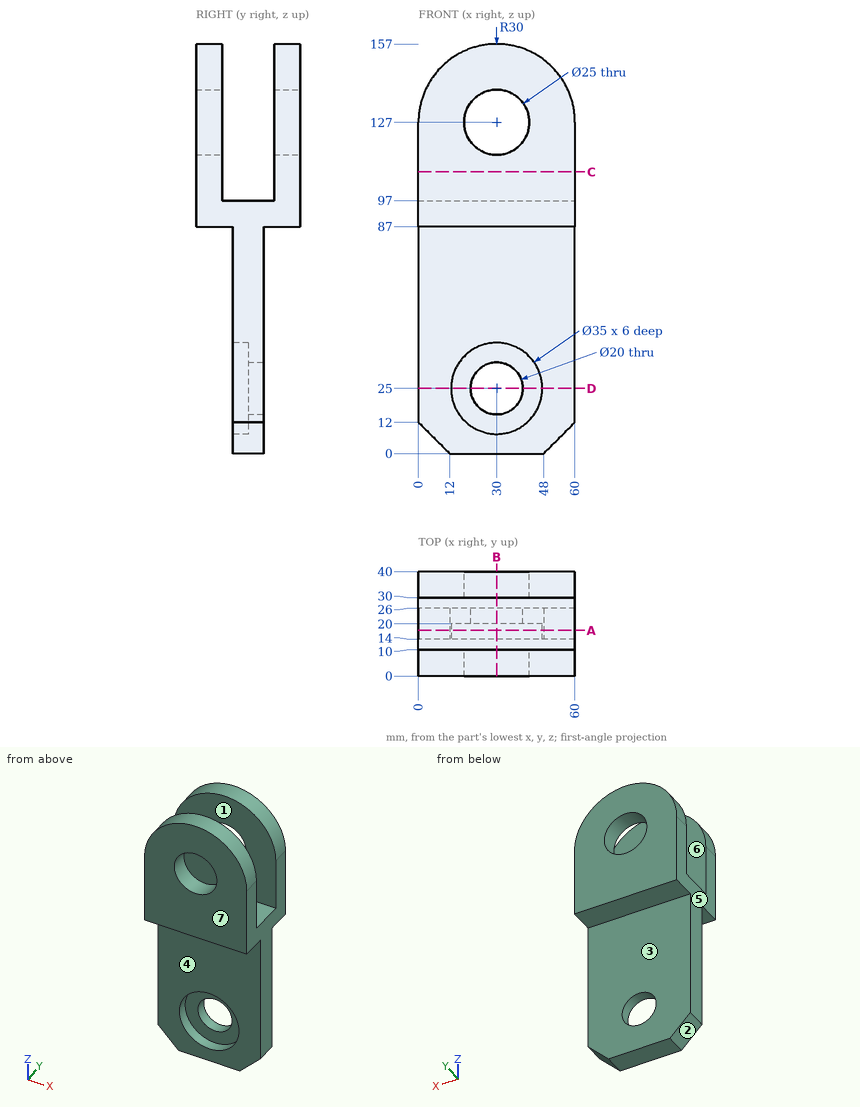
Could you check a few things on this drawing? It's one solid part, dimensions in mm from its lowest x, y, z. A direction names the side the tool comes from. Give positions to 0.01 mm unless a question says otherwise; leave off trailing zeros. Loops run counter-clockwise (first coordinate to the right, second up) from the corner with the lowest first, then second, coordinate; pieces in that order, holes last. Notation, with made-up numbers: (30.5, 6) -> (71.5, 6) arc R27 ccw to (71.5, 24) -> close; hole circle Ø11 at (47.5, 22). An arc over 180 degrees is marked (long way). Use one line per item in the form item = value. Start each with the question number.
1) For P1, Ø8, axis at x = 49.5, y = 33, coming from the +Z side; P2, Ø11, axis at x = 20, y = 5.5, coming from the -Z side; P3, Ø4, axis at x = 26.5, y = 6.5, coming from the +Z side, each with a flat end and sliding along its axis, tell me the tip position at first contact or that it passes through.
2) Thinking about a two-plate mould opening in Y: for the marked faces 5, 6 and 7, which applies, +Y half, -Y half, draft (parallel to the pull), parting line (faces both ways), or undercut?
3) Please list where these lines run through material, in increasing order: line 1 along X through (y, z) = (21, 25); line 2 along Y through (x, z) = (41.5, 97.5); line 3 along X through (y, z) = (7, 127).
4) Imagine slicing it at A-A (y = 17.5). Please give me the cut outline in (x, z).
5) Which directions (+Z, -Z, +X, -X, +Y, -Y) give clear straight access to the entire face, cutting with the end or side of a thin tool? Please do the marked faces 1, 2, 3 and 4.
6) Imagine slicing it at B-B (x = 30). Please give me the cut outline in (y, z).
7) Imagine slicing it at C-C (z = 108). Please give me the cut outline in (x, y), then the cut area to 3 significant figures.
8) Imagine slicing it at D-D (z = 25). Please give me the cut outline in (x, y).
Check values:
q1.P1 = 152.69
q1.P2 = 87
q1.P3 = 156.96
q2.face_5 = draft
q2.face_6 = undercut
q2.face_7 = -Y half
q3.line_1 = 0 to 20, 40 to 60
q3.line_2 = 0 to 10, 30 to 40
q3.line_3 = 0 to 17.5, 42.5 to 60
q4.outline = (0, 12) -> (12, 0) -> (48, 0) -> (60, 12) -> (60, 97) -> (0, 97) -> close; hole circle Ø35 at (30, 25)
q5.face_1 = +Z, +X, -X
q5.face_2 = -Z, -X, +Y, -Y
q5.face_3 = -Z, +X, -X, +Y
q5.face_4 = -Z, +X, -X, -Y
q6.outline = (0, 87) -> (14, 87) -> (14, 42.5) -> (20, 42.5) -> (20, 35) -> (26, 35) -> (26, 87) -> (40, 87) -> (40, 114.5) -> (30, 114.5) -> (30, 97) -> (10, 97) -> (10, 114.5) -> (0, 114.5) -> close; (0, 139.5) -> (10, 139.5) -> (10, 157) -> (0, 157) -> close; (14, 0) -> (26, 0) -> (26, 15) -> (20, 15) -> (20, 7.5) -> (14, 7.5) -> close; (30, 139.5) -> (40, 139.5) -> (40, 157) -> (30, 157) -> close
q7.outline = (0, 0) -> (60, 0) -> (60, 10) -> (0, 10) -> close; (0, 30) -> (60, 30) -> (60, 40) -> (0, 40) -> close
q7.area = 1,200 mm^2
q8.outline = (0, 14) -> (12.5, 14) -> (12.5, 20) -> (20, 20) -> (20, 26) -> (0, 26) -> close; (40, 20) -> (47.5, 20) -> (47.5, 14) -> (60, 14) -> (60, 26) -> (40, 26) -> close
